For this review, take the finished solid that the model builds, in its own axes (mm). Coordinates: 2 decimals unless noted, no trailing zeros. Loops run counter-clockwise (first coordinate to the right, second up) from the corner with the lowest first, then second, coordinate; pieces in that order, holes last. Notation, with made-up numbers: (48, 55.5) -> (82, 55.5) arc R22 cw to (82, 77.5) -> close; hole circle Ø8 at (66, 12). An arc over 180 degrees is marked (long way). Answer in a Markdown table with one row per item.
from build123d import *

# Parameters (mm, degrees)
F0_W     = 200
F0_H     = 60
F1_DEPTH = 10
F3_D     = 32
F5_D     = 5


with BuildPart() as f1:
    # F0 (on Top) → F1 (new body)
    with BuildSketch(Plane.XY):
        with Locations((100, 30)):
            Rectangle(F0_W, F0_H)
    extrude(amount=F1_DEPTH)

    # F3 (through all)
    with Locations(Plane.XY.offset(10)):
        with Locations((102.5, 30), (22.5, 30)):
            Hole(F3_D / 2)

    # F5 (through all)
    with Locations(Plane.XY.offset(10)):
        with Locations((55, 30), (180, 30)):
            Hole(F5_D / 2)


solid = f1.part
Item 1: Insertion check: pin 1 (4 mm diameter, centred on x = 90, y = 24, fed in from +Z); pin 2 (8 mm diameter, centred on x = 180, y = 30, fed in from +Z). Each pin has a flat end and moves straight along its axis. Give the tip position at first contact, or say it passes through.
Worked answers:
| item | result |
|---|---|
| pin 1 | through |
| pin 2 | z = 10 |
Item 2: Take a section at D-D, the plane y = 22. State the section outline as (x, z) points, and give its area (3 significant figures).
Worked answers:
| item | result |
|---|---|
| outline | (0, 0) -> (8.64, 0) -> (8.64, 10) -> (0, 10) -> close; (36.36, 0) -> (88.64, 0) -> (88.64, 10) -> (36.36, 10) -> close; (116.36, 0) -> (200, 0) -> (200, 10) -> (116.36, 10) -> close |
| area | 1,450 mm² |
Item 3: For L1, parallel to X at y = 31, z = 0.75; L2, parallel to Y at x = 22.5, z = 4.5; L3, parallel to X at y = 17, z = 1.5, list the stretches that pass through material, from the lowest coordinate up.
Worked answers:
| item | result |
|---|---|
| L1 | 0 to 6.53, 38.47 to 52.71, 57.29 to 86.53, 118.47 to 177.71, 182.29 to 200 |
| L2 | 0 to 14, 46 to 60 |
| L3 | 0 to 13.17, 31.83 to 93.17, 111.83 to 200 |
Item 4: The part is to be moulded in two halves that separate along Y. For faces 1 (the cylindrical face through (25.97, 14.38, 4.93)), 2 (the flat face through (99, 60, 5)), 3 (the flat face through (200, 30, 5)), say which applies: +Y half, -Y half, draft (parallel to the pull), parting line (faces both ways), or undercut.
Worked answers:
| item | result |
|---|---|
| face 1 | undercut |
| face 2 | +Y half |
| face 3 | draft |
Item 5: Take a section at B-B, the plane y = 30. State the section outline as (x, z) points, and give its area (3 significant figures).
Worked answers:
| item | result |
|---|---|
| outline | (0, 0) -> (6.5, 0) -> (6.5, 10) -> (0, 10) -> close; (38.5, 0) -> (52.5, 0) -> (52.5, 10) -> (38.5, 10) -> close; (57.5, 0) -> (86.5, 0) -> (86.5, 10) -> (57.5, 10) -> close; (118.5, 0) -> (177.5, 0) -> (177.5, 10) -> (118.5, 10) -> close; (182.5, 0) -> (200, 0) -> (200, 10) -> (182.5, 10) -> close |
| area | 1,260 mm² |
Item 6: Take a section at C-C, the plane x = 55. State the section outline as (y, z) points, and give its area (3 significant figures).
Worked answers:
| item | result |
|---|---|
| outline | (0, 0) -> (27.5, 0) -> (27.5, 10) -> (0, 10) -> close; (32.5, 0) -> (60, 0) -> (60, 10) -> (32.5, 10) -> close |
| area | 550 mm² |
Item 7: Take a section at A-A, the plane z = 7. State the section outline as (x, y) points.
Worked answers:
| item | result |
|---|---|
| outline | (0, 0) -> (200, 0) -> (200, 60) -> (0, 60) -> close; hole circle Ø32 at (22.5, 30); hole circle Ø5 at (55, 30); hole circle Ø32 at (102.5, 30); hole circle Ø5 at (180, 30) |
